```python
from build123d import *

# Parameters (mm, degrees)
SKETCH_1_W      = 50
SKETCH_1_H      = 51
SKETCH_1_R      = 9
SKETCH_1_R_2    = 2
SKETCH_1_R_3    = 2.5
EXTRUDE_1_DEPTH = 3
SKETCH_2_W      = 16
SKETCH_2_H      = 6
EXTRUDE_2_DEPTH = 3
SKETCH_3_W      = 49
SKETCH_3_H      = 51
SKETCH_3_R      = 1.5
EXTRUDE_3_DEPTH = 4
FILLET_2_R      = 2
FILLET_3_R      = 2
FILLET_4_R      = 2
FILLET_5_R      = 2
FILLET_6_R      = 2
SKETCH_4_W      = 1.818653348
SKETCH_4_H      = 3.1
EXTRUDE_4_DEPTH = 51


with BuildPart() as part:
    # 草图1 → 凸台-拉伸1 (new body)
    with BuildSketch(Plane.XY):
        with Locations((0, -5.5)):
            Rectangle(SKETCH_1_W, SKETCH_1_H)
        Circle(SKETCH_1_R, mode=Mode.SUBTRACT)
        with Locations((14.5, 0)):
            Circle(SKETCH_1_R_2, mode=Mode.SUBTRACT)
        with Locations((-14.5, 0)):
            Circle(SKETCH_1_R_2, mode=Mode.SUBTRACT)
        with Locations((0, 16)):
            Circle(SKETCH_1_R_3, mode=Mode.SUBTRACT)
        with Locations((0, -16)):
            Circle(SKETCH_1_R_3, mode=Mode.SUBTRACT)
    extrude(amount=EXTRUDE_1_DEPTH)

    # 草图2 → 凸台-拉伸2 (add)
    with BuildSketch(Plane.XZ.offset(31)):
        Polygon((-25, 3), (-25, 106), (24, 106), (25, 3), align=None)
        with Locations((-13.25, 39.5)):
            Rectangle(SKETCH_2_W, SKETCH_2_H, mode=Mode.SUBTRACT)
        Polygon((4.866266466, 42.54910809), (4.92451752, 36.549390862), (20.923763461, 36.704727007), (20.865512407, 42.704444235), align=None, mode=Mode.SUBTRACT)
        with Locations((-13.25, 69.5)):
            Rectangle(SKETCH_2_W, SKETCH_2_H, mode=Mode.SUBTRACT)
        Polygon((20.865512407, 66.295555765), (20.923763461, 72.295272993), (4.92451752, 72.450609138), (4.866266466, 66.45089191), align=None, mode=Mode.SUBTRACT)
    extrude(amount=-EXTRUDE_2_DEPTH)

    # 草图3 → 凸台-拉伸3 (add)
    with BuildSketch(Plane.XY.offset(106)):
        with Locations((-0.5, -5.5)):
            Rectangle(SKETCH_3_W, SKETCH_3_H)
        with Locations((-14.5, 0)):
            Circle(SKETCH_3_R, mode=Mode.SUBTRACT)
        with Locations((14.5, 0)):
            Circle(SKETCH_3_R, mode=Mode.SUBTRACT)
        with Locations((0, -16)):
            Circle(SKETCH_3_R, mode=Mode.SUBTRACT)
        with Locations((0, 16)):
            Circle(SKETCH_3_R, mode=Mode.SUBTRACT)
        with Locations((0, 11.75)):
            Circle(SKETCH_3_R, mode=Mode.SUBTRACT)
    extrude(amount=EXTRUDE_3_DEPTH)

    # 圆角2
    fillet_2_edges = [part.edges().sort_by_distance(p)[0] for p in [
        (-5.25, -29.5, 36.5),
    ]]
    fillet(fillet_2_edges, radius=FILLET_2_R)

    # 圆角3
    fillet_3_edges = [part.edges().sort_by_distance(p)[0] for p in [
        (-21.25, -29.5, 36.5),
        (-21.25, -29.5, 42.5),
        (-5.25, -29.5, 42.5),
    ]]
    fillet(fillet_3_edges, radius=FILLET_3_R)

    # 圆角4
    fillet_4_edges = [part.edges().sort_by_distance(p)[0] for p in [
        (20.865512407, -29.5, 42.704444235),
        (20.923763461, -29.5, 36.704727007),
        (4.92451752, -29.5, 36.549390862),
        (4.866266466, -29.5, 42.54910809),
        (-21.25, -29.5, 66.5),
        (-21.25, -29.5, 72.5),
        (-5.25, -29.5, 72.5),
        (-5.25, -29.5, 66.5),
        (4.866266466, -29.5, 66.45089191),
        (4.92451752, -29.5, 72.450609138),
        (20.923763461, -29.5, 72.295272993),
        (20.865512407, -29.5, 66.295555765),
    ]]
    fillet(fillet_4_edges, radius=FILLET_4_R)

    # 圆角5
    fillet_5_edges = [part.edges().sort_by_distance(p)[0] for p in [
        (0, -28, 3),
    ]]
    fillet(fillet_5_edges, radius=FILLET_5_R)

    # 圆角6
    fillet_6_edges = [part.edges().sort_by_distance(p)[0] for p in [
        (0, -31, 0),
    ]]
    fillet(fillet_6_edges, radius=FILLET_6_R)

    # 草图4 → 凸台-拉伸4 (add)
    with BuildSketch(Plane(origin=(0, -31, 0), x_dir=(-1, 0, 0), z_dir=(0, -1, 0))):
        with Locations((-24.909326674, -108.45)):
            Rectangle(SKETCH_4_W, SKETCH_4_H)
        with Locations((25.909326674, -108.45)):
            Rectangle(SKETCH_4_W, SKETCH_4_H)
    extrude(amount=-EXTRUDE_4_DEPTH)


solid = part.part
```
Geometry check sheet. Reference: the model listing, model coordinates, mm. A direction names the side the tool comes from. Coordinates: 2 decimals unless noted, no trailing zeros. Write each loop counter-clockwise with the first axis right and the second up, starting at its lowest first coordinate (ties: lowest second). Pieces come first, ordered by that corner, then holes. Notation, with made-up numbers: M 66.25,-13 L 78.25,-13 A5 cw 78.25,-5 Z; hole C 15,42 d4. An arc over 180 degrees is marked long. Answer as a JSON object with one key per item and string values.
1. Go/stop test with flat-tipped pins: pin 1 Ø3.5 at (x, y) = (14.5, 0) entering from -Z; pin 2 Ø10 at (x, z) = (20, 29) entering from +Y; pin 3 Ø2.5 at (x, y) = (-14.5, 0) entering from -Z; pin 4 Ø2.5 at (y, z) = (-12, 1) entering from +X. Record where each tip stops, or that it passes through.
Answers below:
{"pin 1": "stops at z = 106", "pin 2": "stops at y = -28", "pin 3": "passes through", "pin 4": "stops at x = 25"}
2. Section check C-C, the plane x = 0. Give the number of separate pieces and of enclosed holes in the cut face, plus the area to 3 significant figures.
Answers below:
{"separate pieces": "7", "enclosed holes": "0", "area": "546 mm²"}
3. Section check A-A, the plane y = -21. Enter the section's corners in (x, z).
Answers below:
{"outline": "M -26.82,106.9 L -25,106.9 L -25,106 L 24,106 L 24,106.9 L 25.82,106.9 L 25.82,110 L -26.82,110 Z; M -25,0 L 25,0 L 25,3 L -25,3 Z"}
4. Section check B-B, the plane x = -14.5. Enter the section's corners in (y, z).
Answers below:
{"outline": "M -31,2 A2 ccw -29,0 L -2,0 L -2,3 L -26,3 A2 cw -28,5 L -28,36.5 L -31,36.5 Z; M -31,42.5 L -28,42.5 L -28,66.5 L -31,66.5 Z; M -31,72.5 L -28,72.5 L -28,106 L -1.5,106 L -1.5,110 L -31,110 Z; M 1.5,106 L 20,106 L 20,110 L 1.5,110 Z; M 2,0 L 20,0 L 20,3 L 2,3 Z"}
5. Scan lines: L1, parallel to Y at x = 0, z = 107.8; L2, parallel to Z at x = 12, y = 9; L3, parallel to Y at x = -14.5, z = 0.7. Record each from-to range of solid material in increasing order.
Answers below:
{"L1": "y = -31 to -17.5, -14.5 to 10.25, 13.25 to 14.5, 17.5 to 20", "L2": "z = 0 to 3, 106 to 110", "L3": "y = -30.52 to -2, 2 to 20"}
6. Draft check along X on faces 5 (the cylindrical face through (-20.65, -29.48, 37.07)), 6 (the flat face through (-6, -8, 3)). Enter one of: released by +X, released by -X, zero draft, split by the parting line, or undercut.
Answers below:
{"face 5": "undercut", "face 6": "zero draft"}
7. Section check D-D, the plane y = 16. Enter the section's corners in (x, z).
Answers below:
{"outline": "M -26.82,106.9 L -25,106.9 L -25,106 L -1.5,106 L -1.5,110 L -26.82,110 Z; M -25,0 L -2.5,0 L -2.5,3 L -25,3 Z; M 1.5,106 L 24,106 L 24,106.9 L 25.82,106.9 L 25.82,110 L 1.5,110 Z; M 2.5,0 L 25,0 L 25,3 L 2.5,3 Z"}
8. Tool access check on faces 1 (the cylindrical face through (-0.325, 10.286, 107.972)), 2 (the cylindrical face through (5.47, -29.48, 41.98)), 3 (the cylindrical face through (-0.325, -17.464, 107.972)), 4 (the cylindrical face through (-0.54, -18.44, 1.48)). Record the directions out of +Z, -Z, +X, -X, +Y, -Y that give a thin tool (end or side, any length) a straight path to the whole face; none if there is none.
Answers below:
{"face 1": "+Z", "face 2": "+Y, -Y", "face 3": "+Z, -Z", "face 4": "-Z"}
